The listing builds one solid part. Answer for the finished solid, in the listing's coordinates (mm). A direction names the side the tool comes from. Give positions to 0.01 mm unless a question says otherwise; leave off trailing zeros. Write each loop counter-clockwise with the first axis right and the second up, starting at its lowest first coordinate (ties: lowest second). Pieces come first, ordered by that corner, then holes. Notation, with made-up numbers: (8.5, 47) -> (38.5, 47) arc R25 ccw to (38.5, 84) -> close; hole circle Ø4 at (87.5, 20). An arc over 180 degrees is marked (long way). Use CSV: the item, a comma, the result in double quotes. Start each with the question number.
from build123d import *

# Parameters (mm, degrees)
SKETCH4_R           = 4
CUT_EXTRUDE1_DEPTH  = 35
SKETCH5_R           = 7
SKETCH5_R_2         = 4
BOSS_EXTRUDE1_DEPTH = 7.5
SKETCH6_R           = 7
SKETCH6_R_2         = 4
BOSS_EXTRUDE3_DEPTH = 5


with BuildPart() as part:
    # Sketch2 → Revolve-Thin7 (revolve)
    with BuildSketch(Plane(origin=(0, 0, 0), x_dir=(0, 0, -1), z_dir=(1, 0, 0)), mode=Mode.PRIVATE) as revolve_thin7_sk:
        with BuildLine():
            Line((0, 5), (-94.77522535, 5))
            ThreePointArc((-94.77522535, 5), (-90.99735594, 18.501939345), (-82.974310102, 30))
            Line((-82.974310102, 30), (-55, 30))
            Line((-55, 30), (-55, 40))
            Line((-55, 40), (-86.90441422, 40))
            ThreePointArc((-86.90441422, 40), (-101.369835612, 19.701900438), (-104.698104926, -5))
            Line((-104.698104926, -5), (0, -5))
            Line((0, -5), (0, 5))
        make_face()
    revolve(revolve_thin7_sk.sketch.rotate(Axis((0, 0, 0), (0, 1, 0)), 180), axis=Axis((0, 0, 0), (0, 1, 0)))

    # Sketch4 → Cut-Extrude1 (cut)
    with BuildSketch(Plane(origin=(0, 5, 0), x_dir=(1, 0, 0), z_dir=(0, 1, 0))):
        with Locations(Location((69.282032303, 0, 0), (0, 0, 90))):
            Circle(SKETCH4_R)
        with Locations(Location((-34.641016151, 60, 0), (0, 0, 90))):
            Circle(SKETCH4_R)
        with Locations(Location((-34.641016151, -60, 0), (0, 0, 90))):
            Circle(SKETCH4_R)
    extrude(amount=CUT_EXTRUDE1_DEPTH, mode=Mode.SUBTRACT)

    # Sketch5 → Boss-Extrude1 (add)
    # profile 1 of 3: a face of its own
    with BuildSketch(Plane(origin=(0, 5, 0), x_dir=(1, 0, 0), z_dir=(0, 1, 0))):
        with Locations(Location((-34.641016151, 60, 0), (0, 0, 270))):
            Circle(SKETCH5_R)
        with Locations(Location((-34.641016151, 60, 0), (0, 0, 90))):
            Circle(SKETCH5_R_2, mode=Mode.SUBTRACT)
    # profile 2 of 3: a face of its own
    with BuildSketch(Plane(origin=(0, 5, 0), x_dir=(1, 0, 0), z_dir=(0, 1, 0))):
        with Locations(Location((-34.641016151, -60, 0), (0, 0, 270))):
            Circle(SKETCH5_R)
        with Locations(Location((-34.641016151, -60, 0), (0, 0, 90))):
            Circle(SKETCH5_R_2, mode=Mode.SUBTRACT)
    # profile 3 of 3: a face of its own
    with BuildSketch(Plane(origin=(0, 5, 0), x_dir=(1, 0, 0), z_dir=(0, 1, 0))):
        with Locations(Location((69.282032303, 0, 0), (0, 0, 270))):
            Circle(SKETCH5_R)
        with Locations(Location((69.282032303, 0, 0), (0, 0, 90))):
            Circle(SKETCH5_R_2, mode=Mode.SUBTRACT)
    extrude(amount=BOSS_EXTRUDE1_DEPTH)

    # Sketch6 → Boss-Extrude3 (add)
    # profile 1 of 3: a face of its own
    with BuildSketch(Plane(origin=(0, 40, 0), x_dir=(1, 0, 0), z_dir=(0, 1, 0))):
        with Locations(Location((-34.641016151, -60, 0), (0, 0, 270))):
            Circle(SKETCH6_R)
        with Locations(Location((-34.641016151, -60, 0), (0, 0, 90))):
            Circle(SKETCH6_R_2, mode=Mode.SUBTRACT)
    # profile 2 of 3: a face of its own
    with BuildSketch(Plane(origin=(0, 40, 0), x_dir=(1, 0, 0), z_dir=(0, 1, 0))):
        with Locations(Location((-34.641016151, 60, 0), (0, 0, 270))):
            Circle(SKETCH6_R)
        with Locations(Location((-34.641016151, 60, 0), (0, 0, 90))):
            Circle(SKETCH6_R_2, mode=Mode.SUBTRACT)
    # profile 3 of 3: a face of its own
    with BuildSketch(Plane(origin=(0, 40, 0), x_dir=(1, 0, 0), z_dir=(0, 1, 0))):
        with Locations(Location((69.282032303, 0, 0), (0, 0, 270))):
            Circle(SKETCH6_R)
        with Locations(Location((69.282032303, 0, 0), (0, 0, 90))):
            Circle(SKETCH6_R_2, mode=Mode.SUBTRACT)
    extrude(amount=BOSS_EXTRUDE3_DEPTH)


solid = part.part
Q1. Section A-A on z = 0 is taken. Give the vertices of the cut face in (x, y).
Q2. Section C-C on y = 35 is taken. Give the vertices of the cut face in (x, z), then the cut area to 3 significant figures.
Q3. Flat-ended cylindrical pins translate along their axes: pin 1 Ø1 at (x, y) = (24, 23) entering from +Z; pin 2 Ø2.5 at (x, z) = (-35.5, 60.5) entering from +Y; pin 3 Ø12 at (x, y) = (-6, 0.5) entering from -Z. Find the tip coordinate at first contact, or state that the pin passes through.
Q4. The mould has two halves that part along Z. Classify faces 1 (the face through (66, 45, 3)), 2 (the face through (65.316, 8.698, 0.521)): +Z half, -Z half, draft (parallel to the pull), parting line (faces both ways), or undercut.
Q5. Section B-B on x = 0 is taken. Give the vertices of the cut face in (y, z).
Q6. Straight lines are drawn through the part: L1, parallel to Y at x = 38.5, z = 61; L2, parallel to X at y = 41.5, z = 60; L3, parallel to Z at x = -34, y = 37.5. For each, find the intervals that lie inside material, in ascending order.
Q7. For faces 3 (the face through (-38, 45, 63)), 4 (the face through (17, 30, -54)), 5 (the face through (-35, 5, -60)), determine the directions among +Z, -Z, +X, -X, +Y, -Y from which every point of the face is accessible in a straight line to the end or side of a thin tool.
Q8. Section D-D on y = 23 is taken. Give the vertices of the cut face in (x, z).
Output:
1,outline,"(-104.7, -5) -> (104.7, -5) arc R51.87 ccw to (86.9, 40) -> (76.28, 40) -> (76.28, 45) -> (73.28, 45) -> (73.28, 30) -> (82.97, 30) arc R41.87 cw to (94.78, 5) -> (76.28, 5) -> (76.28, 12.5) -> (73.28, 12.5) -> (73.28, 5) -> (65.28, 5) -> (65.28, 12.5) -> (62.28, 12.5) -> (62.28, 5) -> (-94.78, 5) arc R41.87 cw to (-82.97, 30) -> (-55, 30) -> (-55, 40) -> (-86.9, 40) arc R51.87 ccw to start; (55, 30) -> (65.28, 30) -> (65.28, 45) -> (62.28, 45) -> (62.28, 40) -> (55, 40) -> close"
2,outline,"circle Ø183.96 at (0, 0); hole circle Ø110 at (0, 0); hole circle Ø8 at (-34.64, -60); hole circle Ø8 at (-34.64, 60); hole circle Ø8 at (69.28, 0)"
2,area,"16,900 mm²"
3,pin 1,"z = 97.28"
3,pin 2,"y = 5"
3,pin 3,"z = -105"
4,face 1,"draft"
4,face 2,"undercut"
5,outline,"(-5, -104.7) arc R51.87 ccw to (40, -86.9) -> (40, -55) -> (30, -55) -> (30, -82.97) arc R41.87 cw to (5, -94.78) -> (5, 94.78) arc R41.87 cw to (30, 82.97) -> (30, 55) -> (40, 55) -> (40, 86.9) arc R51.87 ccw to (-5, 104.7) -> close"
6,L1,"-5 to 5, 30 to 40"
6,L2,"-41.64 to -38.64, -30.64 to -27.64"
6,L3,"-82.92 to -63.95, -56.05 to -43.23, 43.23 to 56.05, 63.95 to 82.92"
7,face 3,"+Z, -Z, +X, -X, +Y"
7,face 4,"none"
7,face 5,"+Y"
8,outline,"circle Ø199.86 at (0, 0); hole circle Ø177.05 at (0, 0)"
